Here's how the part is built. I have some questions about the finished solid (model axes, mm). A direction names the side the tool comes from. Give positions to 0.01 mm unless a question says otherwise; leave off trailing zeros. Loops run counter-clockwise (first coordinate to the right, second up) from the corner with the lowest first, then second, coordinate; pieces in that order, holes last. Notation, with made-up numbers: (-21.75, -8) - (24.25, -8) arc R16 ccw to (24.25, -4) - close; hole circle Ø4 at (53.5, 7). An arc over 180 degrees is marked (long way). Use a Markdown table: item, result.
from build123d import *

# Parameters (mm, degrees)
ESQUISSE1_W                  = 22.3
ESQUISSE1_H                  = 36.68
ESQUISSE1_R                  = 0.7
BOSS_EXTRU_1_DEPTH           = 3
ESQUISSE2_W                  = 11.5
ESQUISSE2_H                  = 4.9
BOSS_EXTRU_2_DEPTH           = 12.3
ESQUISSE3_R                  = 0.7
ENL_V_MAT_EXTRU_1_DEPTH      = 46.571947512
BOSS_EXTRU_3_DEPTH           = 2.1
BOSS_EXTRU_4_DEPTH           = 3
BOSS_EXTRU_5_DEPTH           = 47
ESQUISSE9_W                  = 6.330208048
ESQUISSE9_H                  = 18.044681103
BOSS_EXTRU_6_DEPTH           = 19
BOSS_EXTRU_7_DEPTH           = 5
BOSS_EXTRU_7_DEPTH_BACK      = 11
ENL_V_MAT_EXTRU_3_DEPTH      = 73.539666527
ENL_V_MAT_EXTRU_3_DEPTH_BACK = 73.539666527
ESQUISSE13_R                 = 0.7
ENL_V_MAT_EXTRU_4_DEPTH      = 10
ESQUISSE15_R                 = 2.5
ESQUISSE15_R_2               = 0.7
ENL_V_MAT_EXTRU_5_DEPTH      = 73.212855517
ESQUISSE16_W                 = 11.5
ESQUISSE16_H                 = 4.9
BOSS_EXTRU_8_DEPTH           = 12.3
ESQUISSE17_R                 = 0.7
ENL_V_MAT_EXTRU_6_DEPTH      = 74.831939482
ESQUISSE18_W                 = 7.663831116
ESQUISSE18_H                 = 11.431085426
ENL_V_MAT_EXTRU_7_DEPTH      = 6.3


with BuildPart() as part:
    # Esquisse1 → Boss.-Extru.1 (new body)
    with BuildSketch(Plane.XY):
        with Locations((11.15, 18.34)):
            Rectangle(ESQUISSE1_W, ESQUISSE1_H)
        with Locations((19.8, 32.68)):
            Circle(ESQUISSE1_R, mode=Mode.SUBTRACT)
        with Locations(Location((2.5, 32.68, 0), (0, 0, 180))):
            Circle(ESQUISSE1_R, mode=Mode.SUBTRACT)
        with Locations((2.5, 4)):
            Circle(ESQUISSE1_R, mode=Mode.SUBTRACT)
        with Locations(Location((19.8, 4, 0), (0, 0, 180))):
            Circle(ESQUISSE1_R, mode=Mode.SUBTRACT)
        with Locations((14.8, 32.68)):
            Circle(ESQUISSE1_R, mode=Mode.SUBTRACT)
        with Locations(Location((14.8, 4, 0), (0, 0, 180))):
            Circle(ESQUISSE1_R, mode=Mode.SUBTRACT)
    extrude(amount=BOSS_EXTRU_1_DEPTH)

    # Esquisse2 → Boss.-Extru.2 (add)
    with BuildSketch(Plane(origin=(0, 0, 0), x_dir=(-1, 0, 0), z_dir=(0, 0, -1))):
        with Locations((-16.55, 4.55)):
            Rectangle(ESQUISSE2_W, ESQUISSE2_H)
    extrude(amount=BOSS_EXTRU_2_DEPTH)

    # Esquisse3 → Enlèv. mat.-Extru.1 (cut, through all)
    with BuildSketch(Plane.XY.offset(3)):
        with Locations((14.8, 32.68)):
            Circle(ESQUISSE3_R)
        with Locations((19.8, 32.68)):
            Circle(ESQUISSE3_R)
        with Locations(Location((14.8, 4, 0), (0, 0, 180))):
            Circle(ESQUISSE3_R)
        with Locations(Location((19.8, 4, 0), (0, 0, 180))):
            Circle(ESQUISSE3_R)
    extrude(amount=-ENL_V_MAT_EXTRU_1_DEPTH, mode=Mode.SUBTRACT)

    # Esquisse4 → Boss.-Extru.3 (add)
    with BuildSketch(Plane.XZ.offset(-2.1)):
        Polygon((22.3, 0), (10.844911365, 0), (22.3, -12.182112526), align=None)
    extrude(amount=BOSS_EXTRU_3_DEPTH)

    # Esquisse6 → Boss.-Extru.4 (add)
    with BuildSketch(Plane.XZ):
        with BuildLine():
            Line((14.977510411, 3), (7.322489589, 3))
            Line((7.322489589, 3), (3.441219786, -1.258424259))
            Line((3.441219786, -1.258424259), (1.756159604, -4.536943828))
            Line((1.756159604, -4.536943828), (1.756159604, -7.813164477))
            ThreePointArc((1.756159604, -7.813164477), (11.15, -17.207004873), (20.543840396, -7.813164477))
            Line((20.543840396, -7.813164477), (20.543840396, -4.536943828))
            Line((20.543840396, -4.536943828), (18.858780214, -1.258424259))
            Line((18.858780214, -1.258424259), (14.977510411, 3))
        make_face()
    extrude(amount=BOSS_EXTRU_4_DEPTH)

    # Esquisse8 → Boss.-Extru.5 (add)
    with BuildSketch(Plane.XZ.offset(3)):
        with BuildLine():
            Line((7.984895976, 1.5), (4.684165618, -2.12147208))
            Line((4.684165618, -2.12147208), (3.256159604, -4.89985692))
            Line((3.256159604, -4.89985692), (3.256159604, -7.813164477))
            ThreePointArc((3.256159604, -7.813164477), (11.15, -15.707004873), (19.043840396, -7.813164477))
            Line((19.043840396, -7.813164477), (19.043840396, -4.89985692))
            Line((19.043840396, -4.89985692), (17.615834382, -2.12147208))
            Line((17.615834382, -2.12147208), (14.315104024, 1.5))
            Line((14.315104024, 1.5), (14.315104024, 3))
            Line((14.315104024, 3), (7.984895976, 3))
            Line((7.984895976, 3), (7.984895976, 1.5))
        make_face()
    extrude(amount=BOSS_EXTRU_5_DEPTH)

    # Esquisse9 → Boss.-Extru.6 (add)
    with BuildSketch(Plane.XZ.offset(50)):
        with Locations((11.15, -6.022340552)):
            Rectangle(ESQUISSE9_W, ESQUISSE9_H)
    extrude(amount=BOSS_EXTRU_6_DEPTH)

    # Esquisse10 → Boss.-Extru.7 (add, two sides: drawn at the far end of the back side and taken through both)
    with BuildSketch(Plane.ZY.offset(-7.984895976).offset(-BOSS_EXTRU_7_DEPTH_BACK)):
        with BuildLine():
            Line((3, -62.691900244), (3, -56.361692197))
            Line((3, -56.361692197), (1.5, -56.361692197))
            Line((1.5, -56.361692197), (-2.12147208, -53.060961839))
            Line((-2.12147208, -53.060961839), (-4.89985692, -51.632955825))
            Line((-4.89985692, -51.632955825), (-7.813164477, -51.632955825))
            ThreePointArc((-7.813164477, -51.632955825), (-12.133343304, -52.92007456), (-15.044681103, -56.361692197))
            Line((-15.044681103, -56.361692197), (-15.044681103, -62.691900244))
            ThreePointArc((-15.044681103, -62.691900244), (-12.133343304, -66.133517881), (-7.813164477, -67.420636616))
            Line((-7.813164477, -67.420636616), (-4.89985692, -67.420636616))
            Line((-4.89985692, -67.420636616), (-2.12147208, -65.992630602))
            Line((-2.12147208, -65.992630602), (1.5, -62.691900244))
            Line((1.5, -62.691900244), (3, -62.691900244))
        make_face()
    extrude(amount=BOSS_EXTRU_7_DEPTH + BOSS_EXTRU_7_DEPTH_BACK)

    # Esquisse12 → Enlèv. mat.-Extru.3 (cut, two sides: drawn at the far end of the back side and taken through both)
    with BuildSketch(Plane.ZY.offset(-7.984895976).offset(-ENL_V_MAT_EXTRU_3_DEPTH_BACK)):
        Polygon((-15.044681103, -62.691900244), (-15.044681103, -69), (3, -69), (3, -62.691900244), (1.5, -62.691900244), (-2.12147208, -65.992630602), (-4.89985692, -67.420636616), (-7.813164477, -67.420636616), (-9.686348115, -67.195166272), (-11.232319732, -66.641716708), (-12.800489495, -65.645562875), (-14.068080348, -64.342265423), align=None)
    extrude(amount=ENL_V_MAT_EXTRU_3_DEPTH + ENL_V_MAT_EXTRU_3_DEPTH_BACK, mode=Mode.SUBTRACT)

    # Esquisse13 → Enlèv. mat.-Extru.4 (cut)
    with BuildSketch(Plane.XY.offset(3)):
        with Locations((10.984895976, -5.369741895)):
            Circle(ESQUISSE13_R)
        with Locations((10.984895976, -15.369741895)):
            Circle(ESQUISSE13_R)
        with Locations((10.984895976, -25.369741895)):
            Circle(ESQUISSE13_R)
        with Locations((10.984895976, -35.369741895)):
            Circle(ESQUISSE13_R)
        with Locations((10.984895976, -45.369741895)):
            Circle(ESQUISSE13_R)
        with Locations((10.984895976, -55.369741895)):
            Circle(ESQUISSE13_R)
    extrude(amount=-ENL_V_MAT_EXTRU_4_DEPTH, mode=Mode.SUBTRACT)

    # Esquisse15 → Enlèv. mat.-Extru.5 (cut, through all)
    with BuildSketch(Plane.ZY.offset(-2.984895976)):
        with Locations((-7.813164477, -59.526796221)):
            Circle(ESQUISSE15_R)
        with Locations((-7.813164477, -53.526796221)):
            Circle(ESQUISSE15_R_2)
        with Locations((-2.617012055, -56.526796221)):
            Circle(ESQUISSE15_R_2)
        with Locations((-2.617012055, -62.526796221)):
            Circle(ESQUISSE15_R_2)
        with Locations((-7.813164477, -65.526796221)):
            Circle(ESQUISSE15_R_2)
        with Locations((-13.0093169, -62.526796221)):
            Circle(ESQUISSE15_R_2)
        with Locations((-13.0093169, -56.526796221)):
            Circle(ESQUISSE15_R_2)
    extrude(amount=-ENL_V_MAT_EXTRU_5_DEPTH, mode=Mode.SUBTRACT)

    # Esquisse16 → Boss.-Extru.8 (add)
    with BuildSketch(Plane(origin=(0, 0, 0), x_dir=(-1, 0, 0), z_dir=(0, 0, -1))):
        with Locations((-16.55, 32.23)):
            Rectangle(ESQUISSE16_W, ESQUISSE16_H)
    extrude(amount=BOSS_EXTRU_8_DEPTH)

    # Esquisse17 → Enlèv. mat.-Extru.6 (cut, through all)
    with BuildSketch(Plane.XY.offset(3)):
        with Locations(Location((14.8, 32.68, 0), (0, 0, 180))):
            Circle(ESQUISSE17_R)
        with Locations(Location((19.8, 32.68, 0), (0, 0, 180))):
            Circle(ESQUISSE17_R)
    extrude(amount=-ENL_V_MAT_EXTRU_6_DEPTH, mode=Mode.SUBTRACT)

    # Esquisse18 → Enlèv. mat.-Extru.7 (cut)
    with BuildSketch(Plane(origin=(0, 34.68, 0), x_dir=(1, 0, 0), z_dir=(0, 1, 0))):
        with Locations((14.631915558, 6.584457287)):
            Rectangle(ESQUISSE18_W, ESQUISSE18_H)
    extrude(amount=-ENL_V_MAT_EXTRU_7_DEPTH, mode=Mode.SUBTRACT)


solid = part.part
(1) Suppose I cut it at A-A on y = -39.5. Write out the boundary of the cut face in (x, z), plus the area to 3 significant figures.
A:
| item | result |
|---|---|
| outline | (3.26, -7.81) arc R7.89 ccw to (19.04, -7.81) - (19.04, -4.9) - (17.62, -2.12) - (14.32, 1.5) - (14.32, 3) - (7.98, 3) - (7.98, 1.5) - (4.68, -2.12) - (3.26, -4.9) - close |
| area | 228 mm2 |
(2) Suppose I cut it at B-B on x = 5.75. Count the separate pieces of the cut face and the enclosed holes in it, plus the area to 3 significant figures.
A:
| item | result |
|---|---|
| separate pieces | 2 |
| enclosed holes | 7 |
| area | 950 mm2 |
(3) On a 3-axis mill with a long thin cutter (end or side, diameter ignored), from which of +Z, -Z, +X, -X, +Y, -Y can I reach the whole of each face in a straight line? I mean faces 5 (the face through (20.544, -1, -6)), 6 (the face through (10.976, -26.171, -15.705)), 7 (the face through (16.683, -52.357, -3.491)), 8 (the face through (21, 32, -12.3)). Say none if no direction works.
A:
| item | result |
|---|---|
| face 5 | +Z, -Z, +X, -Y |
| face 6 | -Z |
| face 7 | +Z, +X |
| face 8 | -Z, +X, -X, +Y |
(4) We'd pull the mould along Z, two halves only. Please class faces 1 (the face through (6.358, -26.171, -0.285)), 2 (the face through (18.464, 32, -7)), 3 (the face through (10.873, -61.967, -8.355)), 4 (the face through (10.943, -1.479, -17.205)): pulls with the +Z half, pulls with the -Z half, needs draft (parallel to the pull), parting line crosses it, or undercut.
A:
| item | result |
|---|---|
| face 1 | pulls with the +Z half |
| face 2 | needs draft |
| face 3 | undercut |
| face 4 | pulls with the -Z half |
(5) Will these pins go through, and if not, where does the flat tip stop? pin 1 (1.5 mm diameter, centred on x = 17, z = -7, fed in from +Y); pin 2 (10 mm diameter, centred on x = 15, y = -58.5, fed in from -Z); pin 3 (1 mm diameter, centred on x = 5.5, y = -20.5, fed in from +Z).
A:
| item | result |
|---|---|
| pin 1 | y = 7 |
| pin 2 | z = -15.04 |
| pin 3 | z = -0.68 |
(6) If I drill on line 1 (X direction, y = 4, z = -5.75); line 2 (Y direction, x = 2.5, z = 0.6); line 3 (X direction, y = 32.68, z = -7.25), over which ranges is the centre line in solid material (lowest first)?
A:
| item | result |
|---|---|
| line 1 | 10.8 to 14.1, 15.5 to 19.1, 20.5 to 22.3 |
| line 2 | 0 to 3.3, 4.7 to 31.98, 33.38 to 36.68 |
| line 3 | 18.46 to 19.1, 20.5 to 22.3 |
